Could you check a few things on this model? Use its own coordinates, in mm. Give positions to 0.01 mm unless a question says otherwise; leave off trailing zeros. Loops run counter-clockwise (first coordinate to the right, second up) from the corner with the lowest first, then second, coordinate; pieces in that order, holes last. Notation, with made-up numbers: (79.5, -4.75) - (117.5, -4.75) arc R31 ccw to (117.5, 20.25) - close; hole circle Ø7 at (65.25, -0.75). An arc over 180 degrees is marked (long way). One line per item, written item: value. Start each with the question number.
Q1. If I drill on line 1 (Z direction, x = -81.55, y = 1); line 2 (X direction, y = 2.35, z = -53); line 3 (Z direction, x = -43, y = 3.8), over which ranges is the centre line in solid material (lowest first)? Write a range as from..to.
Q2. I want a section at B-B (z = -53). Please give me the cut outline in (x, y).
Q3. I want a section at D-D (z = -63.09). Please give me the cut outline in (x, y).
Q4. I want a section at C-C (y = 3.3). Please give me the cut outline in (x, z).
Q5. I'm going to push flat-ended pins straight in: P1, Ø4, axis at x = -81, z = -55, coming from the -Y side; P2, Ø2.5, axis at x = -31, y = 3, coming from the +Z side. Where does each tip first touch, or does it pass through?
Q6. I want a section at A-A (x = -61.5). Please give me the cut outline in (y, z), then the cut area to 3 significant figures.
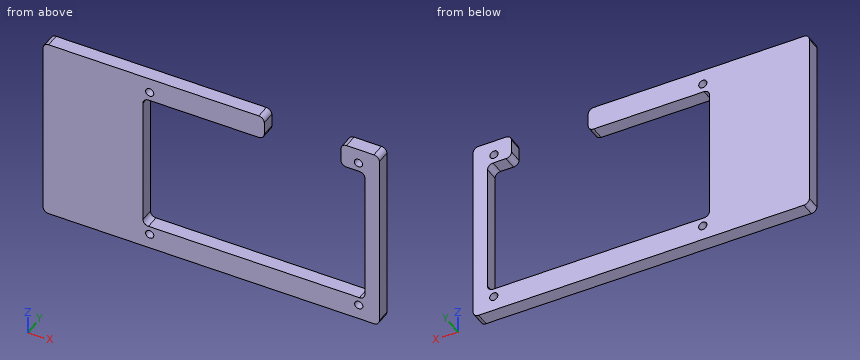
Autodesk Inventor part; units mm, degrees
ref_plane "YZ Plane" through (0, 0, 0) normal (1, 0, 0) x (0, 1, 0)
ref_plane "XZ Plane" through (0, 0, 0) normal (0, 1, 0) x (-1, 0, 0)
ref_plane "XY Plane" through (0, 0, 0) normal (0, 0, 1) x (1, 0, 0)
sketch "Sketch1" plane through (0, 0, 0) normal (0, 1, 0) x (-1, 0, 0)
  line L0 (-2.27, 0) -> (120.44, 0)
  line L1 (120.44, 0) -> (120.44, -68.57)
  line L2 (120.44, -68.57) -> (-2.27, -68.57)
  line L3 (-2.27, -68.57) -> (-2.27, 0)
  line L4 (120.44, -66.57) -> (120.44, -2)
  line L5 (0, -68.57) -> (118.44, -68.57)
  line L6 (-2.27, -2.27) -> (-2.27, -66.3)
  circle A0 centre (81.55, -63.09) radius 1.5
  circle A1 centre (81.55, -63.09) radius 1.5
  line L7 (70.44, -68.57) -> (15.73, -68.57)
  line L8 (51, 0) -> (75, 0)
  line L9 (26, 0) -> (51, 0)
  line L10 (84, -60) -> (79, -60)
  line L11 (79, -60) -> (79, -8.7337)
  line L12 (79, -8.7337) -> (84, -8.7337)
  line L13 (84, -8.7337) -> (84, -60)
  line L14 (8, -60) -> (3, -60)
  line L15 (3, -60) -> (3, -8.7337)
  line L16 (3, -8.7337) -> (8, -8.7337)
  line L17 (8, -8.7337) -> (8, -60)
  circle A2 centre (5.25, -63.09) radius 1.5
  circle A3 centre (5.35, -5.47) radius 1.5
  circle A4 centre (81.55, -5.47) radius 1.5
  circle A5 centre (81.55, -5.47) radius 1.5
  circle A6 centre (5.35, -5.47) radius 1.5
  circle A7 centre (5.25, -63.09) radius 1.5
  dimension "d20" = 3
  dimension "d27" = 3
  dimension "d28" = 3
  dimension "d29" = 3
  dimension "d30" = 68.57
extrude "Extrusion1" add sketch "Sketch1" along normal blind 5
fillet "Fillet4" radius 2 4 edges at (-120.44, 2.5, -68.57) (-120.44, 2.5, 0) (2.27, 2.5, -68.57) (2.27, 2.5, 0)
sketch "Sketch7" plane through (0, 5, 0) normal (0, 1, 0) x (1, 0, 0)
  line L0 (-117.44, 63.57) -> (-87.44, 63.57)
  line L1 (-87.44, 63.57) -> (-87.44, 5)
  line L2 (-87.44, 5) -> (-117.44, 5)
  line L3 (-117.44, 5) -> (-117.44, 63.57)
  line L4 (-120.44, 66.57) -> (-120.44, 2)
  line L5 (0.27, 68.57) -> (-118.44, 68.57)
  line L6 (-118.44, 0) -> (0.27, 0)
  point P0 (0, 0)
  dimension "d67" = 30
  dimension "d68" = 3
  dimension "d69" = 5
  dimension "d70" = 5
extrude "Extrusion6" [suppressed]
fillet "Fillet8" [suppressed]
sketch "Sketch8" plane through (0, 5, 0) normal (0, 1, 0) x (1, 0, 0)
  line L0 (-79, 60) -> (-8, 60)
  line L1 (-8, 60) -> (-8, 8.7337)
  line L2 (-8, 8.7337) -> (-79, 8.7337)
  line L3 (-79, 8.7337) -> (-79, 60)
  line L4 (-8, 8.7337) -> (-8, 60)
  line L5 (0.27, 68.57) -> (-118.44, 68.57)
  line L6 (-79, 60) -> (-79, 8.7337)
  line L7 (-3, 8.7337) -> (-8, 8.7337)
  line L8 (-8, 60) -> (-3, 60)
  point P0 (0, 0)
extrude "Extrusion7" cut sketch "Sketch8" against normal blind 10
sketch "Sketch9" plane through (0, 5, 0) normal (0, 1, 0) x (1, 0, 0)
  line L0 (-3, 8.7337) -> (-84, 8.7337)
  line L1 (-118.44, 0) -> (0.27, 0)
  line L2 (-39.73, 8.7337) -> (-11.73, 8.7337)
  line L3 (-11.73, 8.7337) -> (-11.73, 0)
  line L4 (-11.73, 0) -> (-39.73, 0)
  line L5 (-39.73, 0) -> (-39.73, 8.7337)
  line L6 (2.27, 2) -> (2.27, 66.57)
  point P0 (0, 0)
  point P1 (-79, 8.57)
  point P2 (-8, 8.57)
  point P3 (-39.73, 0)
  point P4 (-11.73, 8.57)
  point P5 (-11.73, 8.7337)
  point P6 (-79, 8.871)
  point P7 (-8, 8.871)
  point P8 (-11.73, 8.871)
  point P9 (-11.73, 8.7337)
  dimension "d78" = 28
  dimension "d81" = 14
  dimension "d82" = 8.7338
extrude "Extrusion8" cut sketch "Sketch9" against normal blind 5
fillet "Fillet9" radius 2 8 edges at (-84, 2.5, -60) (-3, 2.5, -60) (-3, 2.5, -8.7337) (-11.73, 2.5, -8.7337) (-11.73, 2.5, 0) (-39.73, 2.5, -8.7337) (-39.73, 2.5, 0) (-84, 2.5, -8.7337)
properties part number "Top PMMA"
Worked answers:
1. line 1: z = -68.57..-64.59, -61.59..-60, -8.73..-6.97, -3.97..0
1. line 2: x = -120.44..-84, -3..2.27
1. line 3: z = -68.57..-60, -8.73..0
2. outline: (-120.44, 0) - (-84, 0) - (-84, 5) - (-120.44, 5) - close; (-3, 0) - (2.27, 0) - (2.27, 5) - (-3, 5) - close
3. outline: (-120.44, 0) - (-83.05, 0) - (-83.05, 5) - (-120.44, 5) - close; (-80.05, 0) - (-6.75, 0) - (-6.75, 5) - (-80.05, 5) - close; (-3.75, 0) - (2.27, 0) - (2.27, 5) - (-3.75, 5) - close
4. outline: (-120.44, -66.57) arc R2 ccw to (-118.44, -68.57) - (0.27, -68.57) arc R2 ccw to (2.27, -66.57) - (2.27, -2) arc R2 ccw to (0.27, 0) - (-9.73, 0) arc R2 ccw to (-11.73, -2) - (-11.73, -6.73) arc R2 ccw to (-9.73, -8.73) - (-5, -8.73) arc R2 cw to (-3, -10.73) - (-3, -58) arc R2 cw to (-5, -60) - (-82, -60) arc R2 cw to (-84, -58) - (-84, -10.73) arc R2 cw to (-82, -8.73) - (-41.73, -8.73) arc R2 ccw to (-39.73, -6.73) - (-39.73, -2) arc R2 ccw to (-41.73, 0) - (-118.44, 0) arc R2 ccw to (-120.44, -2) - close; hole circle Ø3 at (-81.55, -63.09); hole circle Ø3 at (-81.55, -5.47); hole circle Ø3 at (-5.35, -5.47); hole circle Ø3 at (-5.25, -63.09)
5. P1: passes through
5. P2: stops at z = -60
6. outline: (0, -68.57) - (5, -68.57) - (5, -60) - (0, -60) - close; (0, -8.73) - (5, -8.73) - (5, 0) - (0, 0) - close
6. area: 86.5 mm²
